For this review, take the finished solid that the model builds, in its own axes (mm). Coordinates: 2 decimals unless noted, no trailing zeros. Order: outer loops, then holes, each group sorted by start corner. A loop starts at its lowest first (then second) coordinate and runs counter-clockwise, first axis right, second up. Notation, with made-up numbers: M 1,17 L 17,17 A21 ccw 17,54 Z; hole C -4,55.25 d3. An arc over 180 degrees is marked long. Use CSV: the item, a comma, the result in double quotes.
```python
from build123d import *

# Parameters (mm, degrees)
F1_DEPTH     = 25
F2_D         = 10
F3_T1_DEPTH  = 48
F3_T3_DEPTH  = 68
F3_T6_ANGLE  = 90
F3_T8_ANGLE  = 90
F3_T10_ANGLE = 90
F3_T12_ANGLE = 90
F3_T14_ANGLE = 90
F3_T16_ANGLE = 90
F3_T18_ANGLE = 90
F3_T20_ANGLE = 90


# Not quite as in the source:
# - a fillet or chamfer that OpenCascade refuses, or shapes differently, is made with other operations: its cross-section is extruded or revolved along the edge and cut away or added


with BuildPart() as f1:
    # F0 (on Top) → F1 (new body)
    with BuildSketch(Plane.XY):
        with BuildLine():
            ThreePointArc((40, 24), (38.2426406871, 28.2426406871), (34, 30))
            Line((34, 30), (-34, 30))
            ThreePointArc((-34, 30), (-38.2426406871, 28.2426406871), (-40, 24))
            Line((-40, 24), (-40, -24))
            ThreePointArc((-40, -24), (-38.2426406871, -28.2426406871), (-34, -30))
            Line((-34, -30), (34, -30))
            ThreePointArc((34, -30), (38.2426406871, -28.2426406871), (40, -24))
            Line((40, -24), (40, 24))
        make_face()
    extrude(amount=F1_DEPTH)

    # F2 (through all)
    with Locations(Plane(origin=(0, 0, 0), x_dir=(1, 0, 0), z_dir=(0, 0, -1))):
        with Locations((-32.1810245514, 0), (33.1866517663, 0)):
            Hole(F2_D / 2)

    # F3: fillet of radius 5 on 16 edges, made by hand

    # F3_s2 → F3_t1 (cut)
    with BuildSketch(Plane.XZ.offset(-24)):
        with BuildLine():
            ThreePointArc((40, 20), (38.5355339059, 23.5355339059), (35, 25))
            Line((35, 25), (40, 25))
            Line((40, 25), (40, 20))
        make_face()
        with BuildLine():
            ThreePointArc((40, 5), (38.5355339059, 1.4644660941), (35, 0))
            Line((35, 0), (40, 0))
            Line((40, 0), (40, 5))
        make_face()
        with BuildLine():
            ThreePointArc((-35, 0), (-38.5355339059, 1.4644660941), (-40, 5))
            Line((-40, 5), (-40, 0))
            Line((-40, 0), (-35, 0))
        make_face()
        with BuildLine():
            ThreePointArc((-35, 25), (-38.5355339059, 23.5355339059), (-40, 20))
            Line((-40, 20), (-40, 25))
            Line((-40, 25), (-35, 25))
        make_face()
    extrude(amount=F3_T1_DEPTH, mode=Mode.SUBTRACT)

    # F3_s4 → F3_t3 (cut)
    with BuildSketch(Plane.YZ.offset(-34)):
        with BuildLine():
            ThreePointArc((-30, 5), (-28.5355339059, 1.4644660941), (-25, 0))
            Line((-25, 0), (-30, 0))
            Line((-30, 0), (-30, 5))
        make_face()
        with BuildLine():
            ThreePointArc((-30, 20), (-28.5355339059, 23.5355339059), (-25, 25))
            Line((-25, 25), (-30, 25))
            Line((-30, 25), (-30, 20))
        make_face()
        with BuildLine():
            ThreePointArc((25, 0), (28.5355339059, 1.4644660941), (30, 5))
            Line((30, 5), (30, 0))
            Line((30, 0), (25, 0))
        make_face()
        with BuildLine():
            ThreePointArc((25, 25), (28.5355339059, 23.5355339059), (30, 20))
            Line((30, 20), (30, 25))
            Line((30, 25), (25, 25))
        make_face()
    extrude(amount=F3_T3_DEPTH, mode=Mode.SUBTRACT)

    # F3_s5 → F3_t6 (revolve, cut)
    with BuildSketch(Plane.YZ.offset(34)):
        with BuildLine():
            ThreePointArc((-30, 5), (-28.5355339059, 1.4644660941), (-25, 0))
            Line((-25, 0), (-30, 0))
            Line((-30, 0), (-30, 5))
        make_face()
    revolve(axis=Axis((34, -24, 0), (0, 0, 1)), revolution_arc=F3_T6_ANGLE, mode=Mode.SUBTRACT)

    # F3_s7 → F3_t8 (revolve, cut)
    with BuildSketch(Plane.YZ.offset(34)):
        with BuildLine():
            ThreePointArc((-30, 20), (-28.5355339059, 23.5355339059), (-25, 25))
            Line((-25, 25), (-30, 25))
            Line((-30, 25), (-30, 20))
        make_face()
    revolve(axis=Axis((34, -24, 25), (0, 0, 1)), revolution_arc=F3_T8_ANGLE, mode=Mode.SUBTRACT)

    # F3_s9 → F3_t10 (revolve, cut)
    with BuildSketch(Plane.XZ.offset(24)):
        with BuildLine():
            ThreePointArc((-35, 0), (-38.5355339059, 1.4644660941), (-40, 5))
            Line((-40, 5), (-40, 0))
            Line((-40, 0), (-35, 0))
        make_face()
    revolve(axis=Axis((-34, -24, 0), (0, 0, 1)), revolution_arc=F3_T10_ANGLE, mode=Mode.SUBTRACT)

    # F3_s11 → F3_t12 (revolve, cut)
    with BuildSketch(Plane.XZ.offset(-24)):
        with BuildLine():
            ThreePointArc((35, 0), (38.5355339059, 1.4644660941), (40, 5))
            Line((40, 5), (40, 0))
            Line((40, 0), (35, 0))
        make_face()
    revolve(axis=Axis((34, 24, 0), (0, 0, 1)), revolution_arc=F3_T12_ANGLE, mode=Mode.SUBTRACT)

    # F3_s13 → F3_t14 (revolve, cut)
    with BuildSketch(Plane.YZ.offset(-34)):
        with BuildLine():
            ThreePointArc((25, 0), (28.5355339059, 1.4644660941), (30, 5))
            Line((30, 5), (30, 0))
            Line((30, 0), (25, 0))
        make_face()
    revolve(axis=Axis((-34, 24, 0), (0, 0, 1)), revolution_arc=F3_T14_ANGLE, mode=Mode.SUBTRACT)

    # F3_s15 → F3_t16 (revolve, cut)
    with BuildSketch(Plane.XZ.offset(24)):
        with BuildLine():
            ThreePointArc((-35, 25), (-38.5355339059, 23.5355339059), (-40, 20))
            Line((-40, 20), (-40, 25))
            Line((-40, 25), (-35, 25))
        make_face()
    revolve(axis=Axis((-34, -24, 25), (0, 0, 1)), revolution_arc=F3_T16_ANGLE, mode=Mode.SUBTRACT)

    # F3_s17 → F3_t18 (revolve, cut)
    with BuildSketch(Plane.XZ.offset(-24)):
        with BuildLine():
            ThreePointArc((35, 25), (38.5355339059, 23.5355339059), (40, 20))
            Line((40, 20), (40, 25))
            Line((40, 25), (35, 25))
        make_face()
    revolve(axis=Axis((34, 24, 25), (0, 0, 1)), revolution_arc=F3_T18_ANGLE, mode=Mode.SUBTRACT)

    # F3_s19 → F3_t20 (revolve, cut)
    with BuildSketch(Plane.YZ.offset(-34)):
        with BuildLine():
            ThreePointArc((25, 25), (28.5355339059, 23.5355339059), (30, 20))
            Line((30, 20), (30, 25))
            Line((30, 25), (25, 25))
        make_face()
    revolve(axis=Axis((-34, 24, 25), (0, 0, 1)), revolution_arc=F3_T20_ANGLE, mode=Mode.SUBTRACT)


solid = f1.part
```
Item 1: Add section A-A on z = 17. State the section outline as (x, y) points.
Solutions:
outline,"M -40,-24 A6 ccw -34,-30 L 34,-30 A6 ccw 40,-24 L 40,24 A6 ccw 34,30 L -34,30 A6 ccw -40,24 Z; hole C -32.18,0 d10; hole C 33.19,0 d10"
Item 2: Add section C-C on z = 23.5. State how many separate pieces and enclosed holes the cut face has, and give its area (3 significant figures).
Solutions:
separate pieces,"1"
enclosed holes,"2"
area,"4,230 mm^2"
Item 3: To check wall thickness, follow line 1 along X through (y, z) = (-3, 21.5); line 2 along X through (y, z) = (-4, 14.75); line 3 along X through (y, z) = (24.5, 11.5). State the ranges of each line that lie inside material, in increasing order. Write a range as [from, to].
Solutions:
line 1,"[-39.77, -36.18], [-28.18, 29.19], [37.19, 39.77]"
line 2,"[-40, -35.18], [-29.18, 30.19], [36.19, 40]"
line 3,"[-39.98, 39.98]"
Item 4: Add section B-B on y = 0. State the section outline as (x, z) points, and give its area (3 significant figures).
Solutions:
outline,"M -40,5 A5 ccw -37.18,0.5 L -37.18,24.5 A5 ccw -40,20 Z; M -27.18,0 L 28.19,0 L 28.19,25 L -27.18,25 Z; M 38.19,1.15 A5 ccw 40,5 L 40,20 A5 ccw 38.19,23.85 Z"
area,"1,480 mm^2"
Item 5: Draft analysis for pull direction Y (two halves, no side actions). For faces 1 (the face through (-38.289, -28.196, 12.395)), 2 (the face through (0, 28, 1)), 3 (the face through (38.18, -0.22, 12.68)), state which applies: released by +Y, released by -Y, zero draft, split by the parting line, or undercut.
Solutions:
face 1,"released by -Y"
face 2,"released by +Y"
face 3,"undercut"
